Read the model definition and answer for the solid it produces. Units are mm, in the model's axes. A direction names the side the tool comes from. Coordinates: 2 decimals unless noted, no trailing zeros. Write each loop counter-clockwise with the first axis right and the second up, starting at its lowest first coordinate (ties: lowest second). Pieces come first, ordered by that corner, then holes.
(1) Given pin 1 (1 mm diameter, centred on x = -4.5, y = 7, fed in from +Z); pin 2 (6 mm diameter, centred on x = -12.87, y = 5.8, fed in from +Z), each flat-ended and moving along its own axis, determine where each tip first touches the part or whether it passes through.
(2) Which of the six approach directions +Z, -Z, +X, -X, +Y, -Y give full straight-line access (tool end or side, diameter ignored) to faces 4 (the cylindrical face through (6.12, 5.59, 0.99)), 5 (the cylindrical face through (-7.278, 8.685, 0.986)), 6 (the cylindrical face through (-5.473, 2.917, 0.986))?
(3) The part is cut by section B-B, the plane x = -2.5. Determine the outline of the cut face in (y, z), and give its area (3 significant figures).
(4) Determine the mould class of faces 1 (the cylindrical face through (-13.96, 0.92, 0.99)), 2 (the cylindrical face through (-5.449, 8.697, 0.986)), 3 (the flat face through (-6, 6, 2)) for opening direction Y: pulls with the +Y half, pulls with the -Y half, needs draft (parallel to the pull), parting line crosses it, or undercut.
(5) Straight lines are drawn through the part: line 1 along X through (y, z) = (6, 0.2); line 2 along X through (y, z) = (4, 1.3); line 3 along X through (y, z) = (1.25, 0.6). For each, find the intervals that lie inside material, in ascending order.
(6) The part is cut by section A-A, the plane y = 6.5. Determine the outline of the cut face in (x, z), and give its area (3 significant figures).
(7) The part is cut by section D-D, the plane y = 10. Determine the outline of the cut face in (x, z).
(8) The part is cut by section C-C, the plane z = 1.45. State how many separate pieces and enclosed holes the cut face has, and give its area (3 significant figures).
```python
from build123d import *

# Parameters (mm, degrees)
F0_R     = 5
F1_DEPTH = 2


with BuildPart() as f1:
    # F0 (on Top) → F1 (new body)
    with BuildSketch(Plane.XY):
        with BuildLine():
            ThreePointArc((-6.377694, 8.470873), (-7.290122, 8.691133), (-8.001579, 9.303398))
            ThreePointArc((-8.001579, 9.303398), (-18.873232, 5.800971), (-8.001579, 2.298544))
            ThreePointArc((-8.001579, 2.298544), (-7.290122, 2.910809), (-6.377694, 3.131069))
            Line((-6.377694, 3.131069), (-6.373447, 3.131069))
            ThreePointArc((-6.373447, 3.131069), (-5.461019, 2.910809), (-4.749562, 2.298544))
            ThreePointArc((-4.749562, 2.298544), (6.122091, 5.800971), (-4.749562, 9.303398))
            ThreePointArc((-4.749562, 9.303398), (-5.461019, 8.691133), (-6.373447, 8.470873))
            Line((-6.373447, 8.470873), (-6.377694, 8.470873))
        make_face()
        with Locations((-12.873232, 5.800971)):
            Circle(F0_R, mode=Mode.SUBTRACT)
        with Locations((0.122091, 5.800971)):
            Circle(F0_R, mode=Mode.SUBTRACT)
    extrude(amount=F1_DEPTH)


solid = f1.part
```
Computed:
1. pin 1: stops at z = 2
1. pin 2: passes through
2. face 4: +Z, -Z
2. face 5: +Z, -Z, +Y
2. face 6: +Z, -Z, -Y
3. outline: (0.4, 0) - (1.54, 0) - (1.54, 2) - (0.4, 2) - close; (10.06, 0) - (11.2, 0) - (11.2, 2) - (10.06, 2) - close
3. area: 4.56 mm2
4. face 1: undercut
4. face 2: pulls with the +Y half
4. face 3: needs draft
5. line 1: x = -18.87 to -17.87, -7.88 to -4.87, 5.12 to 6.12
5. line 2: x = -18.6 to -17.54, -8.21 to -4.54, 4.79 to 5.85
5. line 3: x = -16.78 to -14.94, -10.8 to -8.96, -3.79 to -1.95, 2.19 to 4.03
6. outline: (-18.83, 0) - (-17.82, 0) - (-17.82, 2) - (-18.83, 2) - close; (-7.92, 0) - (-4.83, 0) - (-4.83, 2) - (-7.92, 2) - close; (5.07, 0) - (6.08, 0) - (6.08, 2) - (5.07, 2) - close
6. area: 10.2 mm2
7. outline: (-17.16, 0) - (-15.59, 0) - (-15.59, 2) - (-17.16, 2) - close; (-10.16, 0) - (-8.59, 0) - (-8.59, 2) - (-10.16, 2) - close; (-4.16, 0) - (-2.59, 0) - (-2.59, 2) - (-4.16, 2) - close; (2.84, 0) - (4.41, 0) - (4.41, 2) - (2.84, 2) - close
8. separate pieces: 1
8. enclosed holes: 2
8. area: 77.3 mm2
